Verification items for this drawing (mm, ordinates from the low corner). A direction names the side the tool comes from. Give positions to 0.01 mm unless a question says otherwise; leave off trailing zeros. Write each loop counter-clockwise with the first axis right and the second up, starting at its lowest first coordinate (ties: lowest second). Pieces come first, ordered by that corner, then holes. Notation, with made-up numbers: (77, 78) -> (132, 78) arc R16 ccw to (132, 91) -> close; hole circle Ø11 at (-4.5, 49.25). An arc over 180 degrees is marked (long way). One line per item, written item: value.
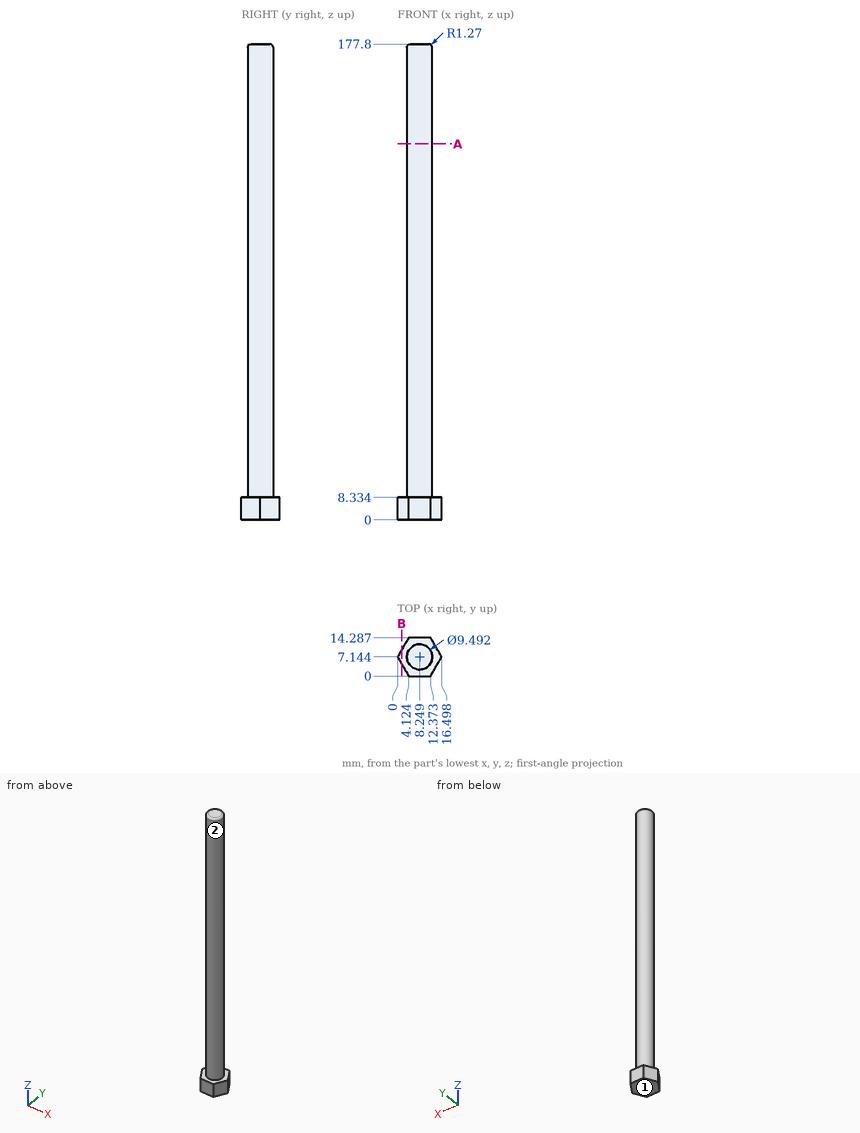
1) Scan lines: probe 1 along Z at (x, y) = (3, 10.5) (1 decimal); probe 2 along Z at (x, y) = (11.5, 8.75); probe 3 along X at (y, z) = (7.5, 139.5). Record each from-to range of solid material in increasing order.
Verdict:
probe 1: 0 to 8.3
probe 2: 0 to 177.79
probe 3: 3.52 to 12.98
2) Sectioned sample at A-A on z = 140.5. Record the cut outline in (x, y) (1 decimal).
Verdict:
outline: circle Ø9.5 at (8.2, 7.1)
3) Sectioned sample at B-B on x = 1.5. Record the cut outline in (y, z) (1 decimal), plus the area to 3 significant figures.
Verdict:
outline: (4.5, 0) -> (9.7, 0) -> (9.7, 8.3) -> (4.5, 8.3) -> close
area: 43.3 mm^2
4) Tool access check on the marked faces 1 and 2. Record the directions out of +Z, -Z, +X, -X, +Y, -Y that give a thin tool (end or side, any length) a straight path to the whole face; none if there is none.
Verdict:
face 1: -Z, +X, -X, +Y, -Y
face 2: +Z
5) Depth check by flat-ended pin: pin 1 Ø4 at (y, z) = (11, 42) entering from +X; pin 2 Ø4 at (x, z) = (10, 74) entering from -Y; pin 3 Ø4 at (y, z) = (9, 20.5) entering from +X (1 decimal). Enter the tip coordinate at first touch or a pass-through.
Verdict:
pin 1: x = 12.62
pin 2: y = 2.4
pin 3: x = 13
